Can you work these out from the drawing? Everything is in mm from the part's minimum corner. A direction names the side the tool comes from. Give positions to 0.01 mm unless a question says otherwise; leave off trailing zeros. Order: outer loops, then holes, each group sorted by start corner. A loop starts at its lowest first (then second) coordinate and runs counter-clockwise, first axis right, second up. Notation, with made-up numbers: (42.5, 47) - (91.5, 47) arc R15 cw to (91.5, 57) - close; hole circle Ø5 at (23.5, 3). An arc over 180 degrees is marked (long way). One line per question, with ' | ' between items.
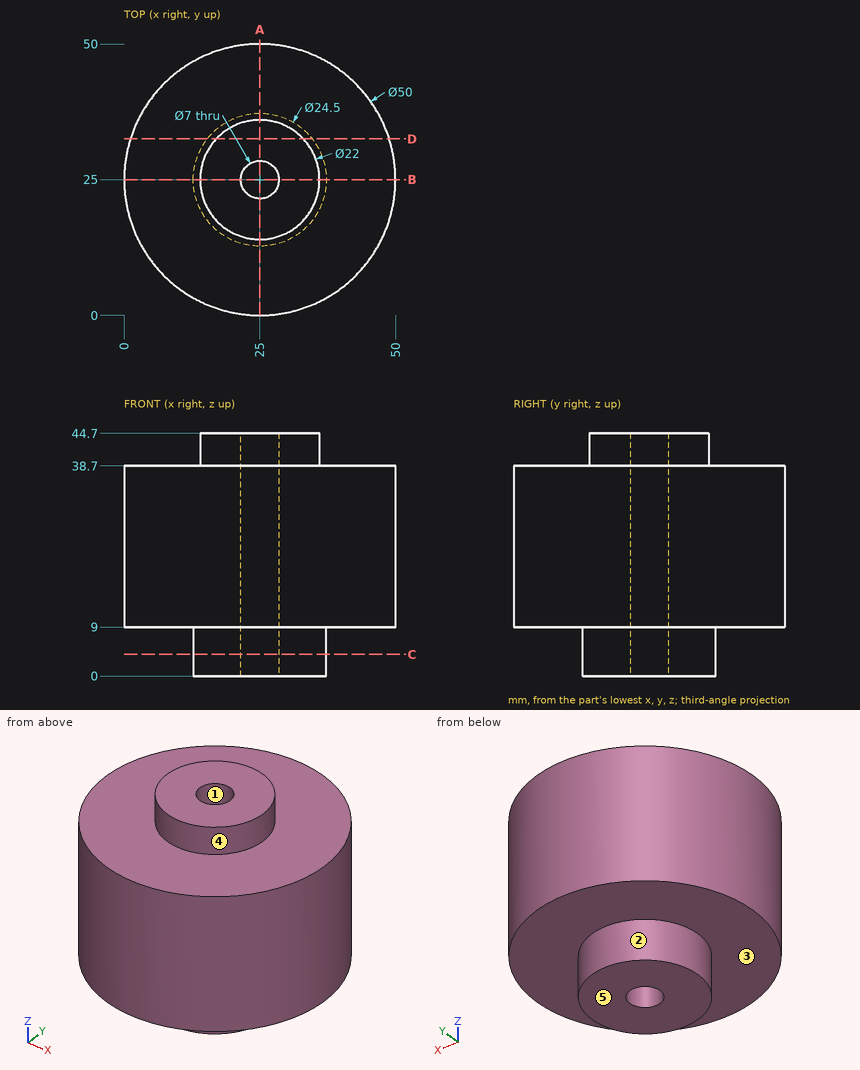
(1) Imagine slicing it at C-C (z = 4). List the corners of the cut face in (x, y) for me.
Answer below:
outline: circle Ø24.5 at (25, 25); hole circle Ø7 at (25, 25)
(2) Imagine slicing it at A-A (x = 25). List the corners of the cut face in (y, z) for me.
Answer below:
outline: (0, 9) - (12.75, 9) - (12.75, 0) - (21.5, 0) - (21.5, 44.7) - (14, 44.7) - (14, 38.7) - (0, 38.7) - close; (28.5, 0) - (37.25, 0) - (37.25, 9) - (50, 9) - (50, 38.7) - (36, 38.7) - (36, 44.7) - (28.5, 44.7) - close
(3) Imagine slicing it at D-D (y = 32.5). List the corners of the cut face in (x, z) for me, and give its area (3 significant figures).
Answer below:
outline: (1.15, 9) - (15.31, 9) - (15.31, 0) - (34.69, 0) - (34.69, 9) - (48.85, 9) - (48.85, 38.7) - (33.05, 38.7) - (33.05, 44.7) - (16.95, 44.7) - (16.95, 38.7) - (1.15, 38.7) - close | area: 1,690 mm^2
(4) Will these pins go through, and if not, where does the flat tip stop? pin 1 (10 mm diameter, centred on y = 31, z = 32, fed in from -X); pin 2 (2 mm diameter, centred on x = 20, y = 37.5, fed in from -Z); pin 3 (12 mm diameter, centred on y = 42.5, z = 25, fed in from -X).
Answer below:
pin 1: x = 0.02 | pin 2: z = 9 | pin 3: x = 2.8
(5) If I drill on line 1 (Y direction, x = 25, z = 12.5); line 2 (Z direction, x = 38, y = 17); line 3 (X direction, y = 26.5, z = 40.5), over which ranges is the centre line in solid material (lowest first)?
Answer below:
line 1: 0 to 21.5, 28.5 to 50 | line 2: 9 to 38.7 | line 3: 14.1 to 21.84, 28.16 to 35.9
(6) If we mould it in two halves opening along Y, with no side actions, what happens to the marked faces 1, 2 and 3? For each: released by +Y, released by -Y, zero draft, split by the parting line, or undercut.
Answer below:
face 1: undercut | face 2: split by the parting line | face 3: zero draft
(7) On a 3-axis mill with a long thin cutter (end or side, diameter ignored), from which of +Z, -Z, +X, -X, +Y, -Y can I reach the whole of each face in a straight line? I mean the marked faces 4 and 5. Say none if no direction works.
Answer below:
face 4: +Z | face 5: -Z, +X, -X, +Y, -Y
